Build history of the part. All positions in model axes, mm. A direction names the side the tool comes from. Round coordinates to 2 decimals unless told otherwise and drop trailing zeros. Order: outer loops, then holes, each group sorted by start corner. A loop starts at its lowest first (then second) coordinate and runs counter-clockwise, first axis right, second up. Notation, with made-up numbers: (15, 0.25) - (23, 0.25) arc R29 ccw to (23, 24.25) - close; hole circle Ø7 at (59, 83). An arc over 180 degrees is marked (long way). Write each question's results on one line, items separated by ' | '. Start each with the question number.
```python
from build123d import *

# Parameters (mm, degrees)
SKETCH1_R           = 12.7
BOSS_EXTRUDE1_DEPTH = 2.54
SKETCH2_R           = 6.35
BOSS_EXTRUDE2_DEPTH = 19.05


with BuildPart() as part:
    # Sketch1 → Boss-Extrude1 (new body)
    with BuildSketch(Plane(origin=(0, 0, 0), x_dir=(0, 0, -1), z_dir=(1, 0, 0))):
        Circle(SKETCH1_R)
    extrude(amount=BOSS_EXTRUDE1_DEPTH)

    # Sketch2 → Boss-Extrude2 (add)
    with BuildSketch(Plane(origin=(2.54, 0, 0), x_dir=(0, 0, -1), z_dir=(1, 0, 0))):
        with Locations(Location((0, 0, 0), (0, 0, 180))):
            Circle(SKETCH2_R)
    extrude(amount=BOSS_EXTRUDE2_DEPTH)

    # Cut-Loft1: read off the stored shape, not the designer's step
    # Cut-Loft1: loft between two sections, ruled curve by curve
    cut_loft1_from = [
        Edge.make_bspline([(0, -0.087914937, -3.173782596), (0, 6.259650254, -3.34961247), (0, 6.435480128, 2.997952721), (0, 0.087914937, 3.173782596), (0, -6.259650254, 3.34961247), (0, -6.435480128, -2.997952721), (0, -0.087914937, -3.173782596)], [0, 0, 0, 0, 0.5, 0.5, 0.5, 1, 1, 1, 1], 3, [1, 0.333333333, 0.333333333, 1, 0.333333333, 0.333333333, 1]),
    ]
    cut_loft1_to = [
        Edge.make_bspline([(21.59, -1.385331043, -4.622892374), (21.59, 7.860453704, -7.393554461), (21.59, 10.631115791, 1.852230287), (21.59, 1.385331043, 4.622892374), (21.59, -7.860453704, 7.393554461), (21.59, -10.631115791, -1.852230287), (21.59, -1.385331043, -4.622892374)], [0, 0, 0, 0, 0.5, 0.5, 0.5, 1, 1, 1, 1], 3, [1, 0.333333333, 0.333333333, 1, 0.333333333, 0.333333333, 1]),
    ]
    cut_loft1 = Solid(Shell([*[Face.make_surface_from_curves(cut_loft1_from[k], cut_loft1_to[k]) for k in range(1)], Face(Wire(cut_loft1_from)), Face(Wire(cut_loft1_to))]))
    add(cut_loft1, mode=Mode.SUBTRACT)


solid = part.part
```
1. Cut at B-B (z = -8). List the corners of the cut face in (x, y).
2. Cut at A-A (y = -9.75). List the corners of the cut face in (x, z), plus the area to 3 significant figures.
3. 3-axis set-ups, long thin cutter, end or side, ignore diameter. For faces 1 (the face through (2.54, 6, -3)), 2 (the face through (1.25, -12.4, 2.75)): which of +Z, -Z, +X, -X, +Y, -Y reach the whole face in a straight line?
4. Flat gauge pins, fed straight in: pin 1 Ø5 at (x, z) = (12.5, 4) entering from +Y; pin 2 Ø5 at (x, z) = (14.5, -6) entering from +Y; pin 3 Ø3 at (x, y) = (9.5, 6.5) entering from -Z. Where does each tip first touch, or does it go through?
5. Wall check: line 1 (X direction, y = 8, z = 1.5); line 2 (Z direction, x = 15.5, y = 0.75); line 3 (Y direction, x = 7, z = -2.25). Give the ranges that are in metal, low to high. Write a range as from..to.
A:
1) outline: (0, -9.86) - (2.54, -9.86) - (2.54, 9.86) - (0, 9.86) - close
2) outline: (0, -8.14) - (2.54, -8.14) - (2.54, 8.14) - (0, 8.14) - close | area: 41.3 mm^2
3) face 1: +X | face 2: +X, -X
4) pin 1: stops at y = 6.17 | pin 2: stops at y = 5.3 | pin 3: stops at z = -3.91
5) line 1: x = 0..2.54 | line 2: z = -6.31..-4.27, 4.27..6.31 | line 3: y = -5.94..-2.91, 2.91..5.94
